from build123d import *

# Parameters (mm, degrees)
SALIENTE_EXTRUIR1_DEPTH = 3
CROQUIS2_R              = 12.5
CROQUIS2_W              = 10
CROQUIS2_H              = 45
CORTAR_EXTRUIR1_DEPTH   = 3
CROQUIS4_R              = 1.75
CORTAR_EXTRUIR2_DEPTH   = 3
CROQUIS5_R              = 1.75
CORTAR_EXTRUIR3_DEPTH   = 3
CROQUIS6_R              = 1.75
CORTAR_EXTRUIR4_DEPTH   = 3
CROQUIS7_R              = 1.5
CORTAR_EXTRUIR5_DEPTH   = 10
CROQUIS8_R              = 1.75
CORTAR_EXTRUIR6_DEPTH   = 10


with BuildPart() as part:
    # Croquis1 → Saliente-Extruir1 (new body)
    with BuildSketch(Plane.XY):
        with BuildLine():
            Line((-41.533119315, 0), (-41.533119315, 50))
            ThreePointArc((-41.533119315, 50), (-58.84153616, 27.616546168), (-65, 0))
            Line((-65, 0), (-41.533119315, 0))
        make_face()
        with BuildLine():
            Line((-41.533119315, -50), (-41.533119315, 0))
            Line((-41.533119315, 0), (-65, 0))
            ThreePointArc((-65, 0), (-58.84153616, -27.616546168), (-41.533119315, -50))
        make_face()
        with BuildLine():
            Line((17.853571071, 0), (-41.533119315, 0))
            Line((-41.533119315, 0), (-41.533119315, -50))
            ThreePointArc((-41.533119315, -50), (-37.997585409, -48.535533906), (-36.533119315, -45))
            Line((-36.533119315, -45), (-36.533119315, -35))
            Line((-36.533119315, -35), (13.466880685, -35))
            Line((13.466880685, -35), (13.466880685, -55))
            ThreePointArc((13.466880685, -55), (14.106925019, -59.658513326), (17.853571071, -62.5))
            Line((17.853571071, -62.5), (17.853571071, 0))
        make_face()
        with BuildLine():
            ThreePointArc((-36.533119315, 45), (-37.997585409, 48.535533906), (-41.533119315, 50))
            Line((-41.533119315, 50), (-41.533119315, 0))
            Line((-41.533119315, 0), (17.853571071, 0))
            Line((17.853571071, 0), (17.853571071, 62.5))
            ThreePointArc((17.853571071, 62.5), (14.106925019, 59.658513326), (13.466880685, 55))
            Line((13.466880685, 55), (13.466880685, 35))
            Line((13.466880685, 35), (-36.533119315, 35))
            Line((-36.533119315, 35), (-36.533119315, 45))
        make_face()
        with BuildLine():
            ThreePointArc((65, 0), (51.891628032, 39.144079248), (17.853571071, 62.5))
            Line((17.853571071, 62.5), (17.853571071, 0))
            Line((17.853571071, 0), (65, 0))
        make_face()
        with BuildLine():
            Line((65, 0), (17.853571071, 0))
            Line((17.853571071, 0), (17.853571071, -62.5))
            ThreePointArc((17.853571071, -62.5), (51.891628032, -39.144079248), (65, 0))
        make_face()
    extrude(amount=SALIENTE_EXTRUIR1_DEPTH)

    # Croquis2 → Cortar-Extruir1 (cut)
    with BuildSketch(Plane.XY.offset(3)):
        Circle(CROQUIS2_R)
        with Locations((-36.533119315, 0)):
            Rectangle(CROQUIS2_W, CROQUIS2_H)
    extrude(amount=-CORTAR_EXTRUIR1_DEPTH, mode=Mode.SUBTRACT)

    # Croquis4 → Cortar-Extruir2 (cut)
    with BuildSketch(Plane.XY.offset(3)):
        with Locations((-53.533119315, 18)):
            Circle(CROQUIS4_R)
        with Locations((-17.533119315, 18)):
            Circle(CROQUIS4_R)
        with Locations(Location((-17.533119315, -18, 0), (0, 0, 180))):
            Circle(CROQUIS4_R)
        with Locations(Location((-53.533119315, -18, 0), (0, 0, 180))):
            Circle(CROQUIS4_R)
    extrude(amount=-CORTAR_EXTRUIR2_DEPTH, mode=Mode.SUBTRACT)

    # Croquis5 → Cortar-Extruir3 (cut)
    with BuildSketch(Plane.XY.offset(3)):
        with Locations((-42, 44)):
            Circle(CROQUIS5_R)
        with Locations((18, 58)):
            Circle(CROQUIS5_R)
        with Locations(Location((18, -58, 0), (0, 0, 180))):
            Circle(CROQUIS5_R)
        with Locations(Location((-42, -44, 0), (0, 0, 180))):
            Circle(CROQUIS5_R)
    extrude(amount=-CORTAR_EXTRUIR3_DEPTH, mode=Mode.SUBTRACT)

    # Croquis6 → Cortar-Extruir4 (cut)
    with BuildSketch(Plane.XY.offset(3)):
        with Locations((6, -15.81)):
            Circle(CROQUIS6_R)
        with Locations((54.4, -17.52)):
            Circle(CROQUIS6_R)
        with Locations((49.4, 35)):
            Circle(CROQUIS6_R)
        with Locations((21.44, 35)):
            Circle(CROQUIS6_R)
    extrude(amount=-CORTAR_EXTRUIR4_DEPTH, mode=Mode.SUBTRACT)

    # Croquis7 → Cortar-Extruir5 (cut)
    with BuildSketch(Plane.XY.offset(3)):
        with Locations((-21.683119315, -30)):
            Circle(CROQUIS7_R)
        with Locations((-1.383119315, -30)):
            Circle(CROQUIS7_R)
        with Locations((-1.383119315, 30)):
            Circle(CROQUIS7_R)
        with Locations((-21.683119315, 30)):
            Circle(CROQUIS7_R)
    extrude(amount=-CORTAR_EXTRUIR5_DEPTH, mode=Mode.SUBTRACT)

    # Croquis8 → Cortar-Extruir6 (cut)
    with BuildSketch(Plane.XY.offset(3)):
        with Locations((59, 19.5)):
            Circle(CROQUIS8_R)
        with Locations((59, -19.5)):
            Circle(CROQUIS8_R)
    extrude(amount=-CORTAR_EXTRUIR6_DEPTH, mode=Mode.SUBTRACT)


solid = part.part
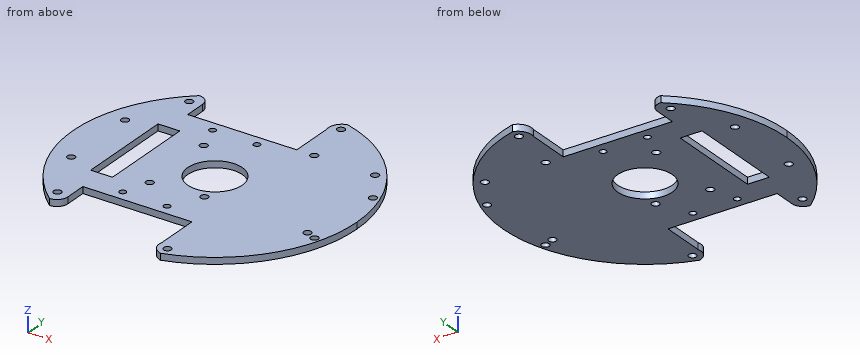
Geometry check sheet. Reference: the model listing, model coordinates, mm. Give positions to 0.01 mm unless a question says otherwise; leave off trailing zeros. Loops run counter-clockwise (first coordinate to the right, second up) from the corner with the lowest first, then second, coordinate; pieces in that order, holes last. Notation, with made-up numbers: M -36,-32 L -30,-32 A22 ccw -30,1 Z; hole C 42.25,-26.75 d10. An arc over 180 degrees is marked long. Answer as a JSON object with one key per item and string values. Group by question number.
Item 1: Gauge pin test, flat ends, axial feed: pin 1 (1.5 mm diameter, centred on y = -10, z = 0.5, fed in from -X); pin 2 (1.5 mm diameter, centred on y = -48.5, z = 1.5, fed in from -X); pin 3 (0.9 mm diameter, centred on y = -39.5, z = 2, fed in from +X). Record the tip position at first contact, or that the pin passes through.
Item 2: Sectioned sample at A-A on x = 10. Record the boundary of the cut face in (y, z).
Item 3: Sectioned sample at B-B on y = 3. Record the boundary of the cut face in (x, z).
Item 4: Material ranges on L1, parallel to Y at x = -21.5, z = 2.15; L2, parallel to Y at x = 18, z = 1.35; L3, parallel to X at y = -29, z = 0.8, recorded low to high.
Item 5: Sectioned sample at C-C on y = -40.5. Record the boundary of the cut face in (x, z), plus the area to 3 significant figures.
Item 6: Sectioned sample at D-D on x = 59. Record the boundary of the cut face in (y, z), plus the area to 3 significant figures.
Findings below:
{
 "1": {"pin 1": "x = -64.34", "pin 2": "x = -44.1", "pin 3": "x = 51.96"},
 "2": {"outline": "M -35,0 L -7.5,0 L -7.5,3 L -35,3 Z; M 7.5,0 L 35,0 L 35,3 L 7.5,3 Z"},
 "3": {"outline": "M -64.93,0 L -41.53,0 L -41.53,3 L -64.93,3 Z; M -31.53,0 L -12.13,0 L -12.13,3 L -31.53,3 Z; M 12.13,0 L 64.93,0 L 64.93,3 L 12.13,3 Z"},
 "4": {"L1": "-35 to -31.49, -28.51 to 28.51, 31.49 to 35", "L2": "-62.46 to -59.75, -56.25 to 56.25, 59.75 to 62.46", "L3": "-58.17 to -22.8, -20.57 to -2.5, -0.27 to 58.17"},
 "5": {"outline": "M -50.84,0 L -36.53,0 L -36.53,3 L -50.84,3 Z; M 13.47,0 L 50.84,0 L 50.84,3 L 13.47,3 Z", "area": "155 mm2"},
 "6": {"outline": "M -27.28,0 L -21.25,0 L -21.25,3 L -27.28,3 Z; M -17.75,0 L 17.75,0 L 17.75,3 L -17.75,3 Z; M 21.25,0 L 27.28,0 L 27.28,3 L 21.25,3 Z", "area": "143 mm2"}
}
